Verification items for the finished model (mm, model axes). A direction names the side the tool comes from. Give positions to 0.01 mm unless a question says otherwise; leave off trailing zeros. Loops run counter-clockwise (first coordinate to the right, second up) from the corner with the lowest first, then second, coordinate; pieces in that order, holes last. Notation, with made-up numbers: M 87.5,43 L 135.5,43 A25 cw 135.5,61 Z; hole C 14.25,61 d11. An arc over 180 degrees is marked long. Use a Markdown table: item, result.
from build123d import *

# Parameters (mm, degrees)
F1_W     = 25.4
F1_H     = 25.4
F1_W_2   = 22.225
F1_H_2   = 22.225
F2_DEPTH = 101.6
F4_D     = 3.175
F6_D     = 3.175


with BuildPart() as f2:
    # F1 (on face) → F2 (new body)
    with BuildSketch(Plane.XY):
        with Locations((21.07109, -27.648601)):
            Rectangle(F1_W, F1_H)
        with Locations((21.086402, -27.549498)):
            Rectangle(F1_W_2, F1_H_2, mode=Mode.SUBTRACT)
    extrude(amount=F2_DEPTH)

    # F4 (through all)
    with Locations(Plane(origin=(0, -14.948601, 0), x_dir=(-1, 0, 0), z_dir=(0, 1, 0))):
        with Locations((-20.819843, 12.163988)):
            Hole(F4_D / 2)

    # F6 (through all)
    with Locations(Plane(origin=(8.37109, 0, 0), x_dir=(0, -1, 0), z_dir=(-1, 0, 0))):
        with Locations((28.359888, 7.072924)):
            Hole(F6_D / 2)


solid = f2.part
(1) Material ranges on line 1 (X direction, y = -26.75, z = 78); line 2 (Y direction, x = 13, z = 16), recorded low to high.
Results below:
| item | result |
|---|---|
| line 1 | 8.37 to 9.97, 32.2 to 33.77 |
| line 2 | -40.35 to -38.66, -16.44 to -14.95 |
(2) Cross-section at C-C on z = 58.5. Record the cut outline in (x, y).
Results below:
| item | result |
|---|---|
| outline | M 8.37,-40.35 L 33.77,-40.35 L 33.77,-14.95 L 8.37,-14.95 Z; hole M 9.97,-38.66 L 32.2,-38.66 L 32.2,-16.44 L 9.97,-16.44 Z |
(3) Gauge pin test, flat end, axial feed: P1, Ø3, axis at y = -28.36, z = 7.07, coming from the +X side. Record the tip position at first contact, or that the pin passes through.
Results below:
| item | result |
|---|---|
| P1 | through |
(4) Cross-section at B-B on y = -19.5. Record the cut outline in (x, z), then the cut area to 3 significant figures.
Results below:
| item | result |
|---|---|
| outline | M 8.37,0 L 9.97,0 L 9.97,101.6 L 8.37,101.6 Z; M 32.2,0 L 33.77,0 L 33.77,101.6 L 32.2,101.6 Z |
| area | 323 mm^2 |
(5) Set-up check for faces 4 (the flat face through (21, -38.662, 50)), 5 (the cylindrical face through (22.334, -39.517, 12.641)): record each of +Z, -Z, +X, -X, +Y, -Y from which the full face is reachable in a straight line by a thin tool's end or side.
Results below:
| item | result |
|---|---|
| face 4 | +Z, -Z |
| face 5 | +Y, -Y |
(6) Draft check along Z on faces 1 (the flat face through (21, -16.437, 50)), 2 (the cylindrical face through (32.996, -27.506, 8.412)), 3 (the flat face through (9.7, -27.6, 0)). Enter one of: +Z half, -Z half, draft (parallel to the pull), parting line (faces both ways), or undercut.
Results below:
| item | result |
|---|---|
| face 1 | draft |
| face 2 | undercut |
| face 3 | -Z half |
(7) Cross-section at A-A on x = 13.25. Record the cut outline in (y, z).
Results below:
| item | result |
|---|---|
| outline | M -40.35,0 L -38.66,0 L -38.66,101.6 L -40.35,101.6 Z; M -16.44,0 L -14.95,0 L -14.95,101.6 L -16.44,101.6 Z |
(8) Cross-section at D-D on y = -28.75. Record the cut outline in (x, z), then the cut area to 3 significant figures.
Results below:
| item | result |
|---|---|
| outline | M 8.37,0 L 9.97,0 L 9.97,5.53 L 8.37,5.53 Z; M 8.37,8.61 L 9.97,8.61 L 9.97,101.6 L 8.37,101.6 Z; M 32.2,0 L 33.77,0 L 33.77,5.53 L 32.2,5.53 Z; M 32.2,8.61 L 33.77,8.61 L 33.77,101.6 L 32.2,101.6 Z |
| area | 313 mm^2 |
